Check sheet for the drawn part. Datum: minimum x, y, z corner. Units: mm. A direction names the side the tool comes from. Coordinates: 2 decimals unless noted, no trailing zeros. Order: outer loops, then holes, each group sorted by start corner. A loop starts at its lowest first (then second) coordinate and runs counter-clockwise, first axis right, second up. Notation, with made-up numbers: (76.25, -38) -> (87.25, -38) arc R31 cw to (87.25, -5) -> close; hole circle Ø4 at (8, -33.5). An arc over 180 degrees is marked (long way). Answer as CSV lines item,"result".
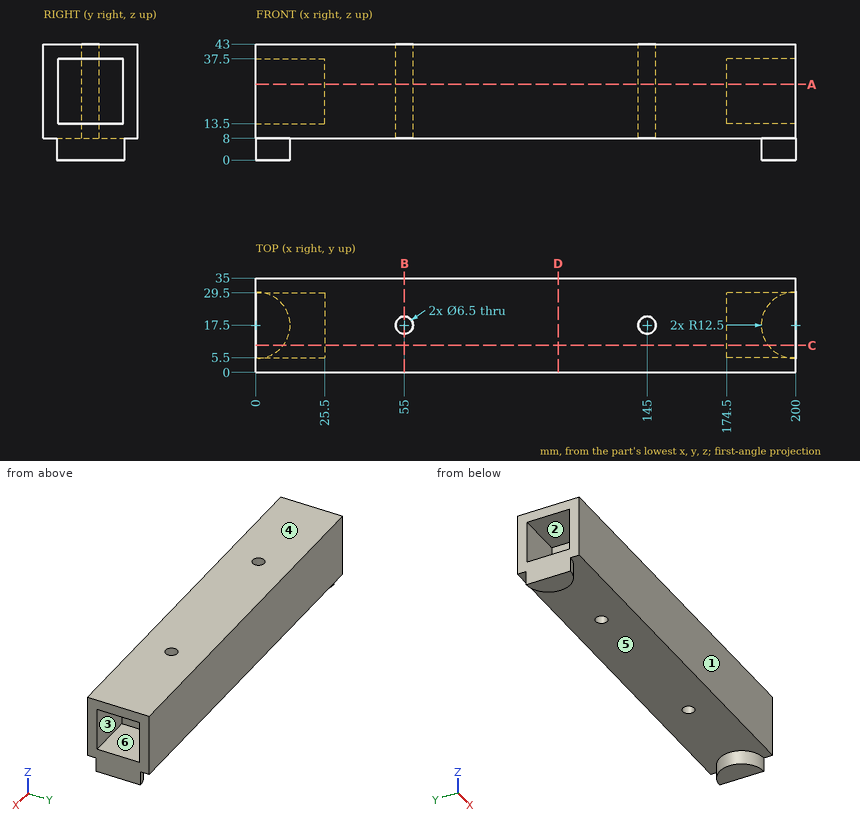
Item 1: Release check for a two-part mould opening along Z. For the marked faces 4, 5 and 6 record: +Z half, -Z half, draft (parallel to the pull), parting line (faces both ways), or undercut.
Answer list:
face 4,"+Z half"
face 5,"-Z half"
face 6,"undercut"
Item 2: Thickness scan on line 1 (X direction, y = 17.5, z = 18.5); line 2 (Z direction, x = 21, y = 29); line 3 (Y direction, x = 55, z = 15). Record the ranges inside material, lowest first.
Answer list:
line 1,"25.5 to 51.75, 58.25 to 141.75, 148.25 to 174.5"
line 2,"8 to 13.5, 37.5 to 43"
line 3,"0 to 14.25, 20.75 to 35"
Item 3: Section check A-A, the plane z = 28. Record the boundary of the cut face in (x, y).
Answer list:
outline,"(0, 0) -> (200, 0) -> (200, 5.5) -> (174.5, 5.5) -> (174.5, 29.5) -> (200, 29.5) -> (200, 35) -> (0, 35) -> (0, 29.5) -> (25.5, 29.5) -> (25.5, 5.5) -> (0, 5.5) -> close; hole circle Ø6.5 at (55, 17.5); hole circle Ø6.5 at (145, 17.5)"
Item 4: Section check B-B, the plane x = 55. Record the boundary of the cut face in (y, z).
Answer list:
outline,"(0, 8) -> (14.25, 8) -> (14.25, 43) -> (0, 43) -> close; (20.75, 8) -> (35, 8) -> (35, 43) -> (20.75, 43) -> close"
Item 5: Tool access check on the marked faces 1, 2 and 3. Record the directions out of +Z, -Z, +X, -X, +Y, -Y that give a thin tool (end or side, any length) a straight path to the whole face; none if there is none.
Answer list:
face 1,"+Z, -Z, +X, -X, -Y"
face 2,"-X"
face 3,"+X"
Item 6: Section check D-D, the plane x = 112. Record the boundary of the cut face in (y, z), plus the area to 4 significant figures.
Answer list:
outline,"(0, 8) -> (35, 8) -> (35, 43) -> (0, 43) -> close"
area,"1,225 mm2"
Item 7: Section check C-C, the plane y = 10. Record the boundary of the cut face in (x, z).
Answer list:
outline,"(0, 0) -> (10, 0) -> (10, 8) -> (190, 8) -> (190, 0) -> (200, 0) -> (200, 13.5) -> (174.5, 13.5) -> (174.5, 37.5) -> (200, 37.5) -> (200, 43) -> (0, 43) -> (0, 37.5) -> (25.5, 37.5) -> (25.5, 13.5) -> (0, 13.5) -> close"
Item 8: Depth check by flat-ended pin: pin 1 Ø4 at (y, z) = (10, 20.5) entering from -X; pin 2 Ø2 at (x, y) = (88.5, 13) entering from -Z; pin 3 Ø8 at (y, z) = (14, 26) entering from +X. Enter the tip coordinate at first touch or a pass-through.
Answer list:
pin 1,"x = 25.5"
pin 2,"z = 8"
pin 3,"x = 174.5"
